The model under review builds one solid part; all positions refer to its coordinate system, in mm. A direction names the side the tool comes from. Round coordinates to 2 decimals unless told otherwise and drop trailing zeros. Order: outer loops, then holes, each group sorted by start corner. A loop starts at its lowest first (then second) coordinate and runs counter-clockwise, first axis right, second up.
Autodesk Inventor part; units mm, degrees
ref_plane "YZ Plane" through (0, 0, 0) normal (1, 0, 0) x (0, 1, 0)
ref_plane "XZ Plane" through (0, 0, 0) normal (0, 1, 0) x (-1, 0, 0)
ref_plane "XY Plane" through (0, 0, 0) normal (0, 0, 1) x (1, 0, 0)
sketch "Sketch1" plane through (0, 0, 0) normal (0, 0, 1) x (1, 0, 0)
  line L0 (-35.56, 0) -> (35.56, 0) construction
  line L1 (0, -35.56) -> (0, 35.56) construction
  line L2 (-25.4, 25.4) -> (25.4, 25.4)
  line L3 (25.4, 25.4) -> (25.4, -25.4)
  line L4 (25.4, -25.4) -> (-25.4, -25.4)
  line L5 (-25.4, -25.4) -> (-25.4, 25.4)
  line L6 (-22.225, 22.225) -> (22.225, 22.225)
  line L7 (22.225, 22.225) -> (22.225, -22.225)
  line L8 (22.225, -22.225) -> (-22.225, -22.225)
  line L9 (-22.225, -22.225) -> (-22.225, 22.225)
  point P0 (0, 0)
  point P1 (-25.4, 0)
  point P2 (0, 25.4)
  point P3 (-22.225, 0)
  point P4 (0, 22.225)
  dimension "d0" = 50.8
  dimension "d1" = 3.175
  dimension "d11" = 50.8
  dimension "d12" = 3.175
extrude "Extrusion1" add sketch "Sketch1" along normal mid plane 101.6
sketch "Sketch6" plane through (-25.4, -25.4, 50.8) normal (-1, 0, 0) x (0, 0, 1)
  circle A0 centre (-68.7605, 43.3605) radius 2.0193 construction
  circle A1 centre (-32.8395, 7.4395) radius 2.0193 construction
  circle A2 centre (-50.8, 25.4) radius 6.985
  line L0 (0, 47.625) -> (-101.6, 47.625) construction
  line L1 (-101.6, 3.175) -> (-101.6, 47.625) construction
  line L2 (0, 3.175) -> (-101.6, 3.175) construction
  line L3 (0, 47.625) -> (0, 3.175) construction
  circle A3 centre (-86.7029, 41.275) radius 3.175
  circle A4 centre (-14.8971, 9.525) radius 3.175
  circle A5 centre (-86.7029, 9.525) radius 3.175
  circle A6 centre (-14.8971, 41.275) radius 3.175
  circle A7 centre (-68.7605, 43.3605) radius 2.413
  circle A8 centre (-32.8395, 7.4395) radius 2.413
  point P0 (-50.8, 25.4)
  dimension "d38" = 4.826
sketch "Sketch7" plane through (25.4, -25.4, 50.8) normal (1, 0, 0) x (0, 0, -1)
  circle A0 centre (50.8, 25.4) radius 14.2875
  dimension "d25" = 28.575
extrude "Extrusion8" cut sketch "Sketch7" against normal up to next
sketch "Sketch8" plane through (-22.225, -22.225, -50.8) normal (1, 0, 0) x (0, 0, -1)
  circle A0 centre (-14.8971, 6.35) radius 2.667
  circle A1 centre (-86.7029, 6.35) radius 2.667
  circle A2 centre (-86.7029, 38.1) radius 2.667
  circle A3 centre (-14.8971, 38.1) radius 2.667
  point P0 (-50.8, 22.225)
extrude "Extrusion9" cut sketch "Sketch8" against normal up to next
sketch "Sketch9" plane through (25.4, -25.4, 50.8) normal (1, 0, 0) x (0, 0, -1)
  circle A0 centre (14.8971, 9.525) radius 3.175
  circle A1 centre (14.8971, 41.275) radius 3.175
  circle A2 centre (86.7029, 9.525) radius 3.175
  circle A3 centre (86.7029, 41.275) radius 3.175
  point P0 (50.8, 25.4)
extrude "Extrusion10" cut sketch "Sketch9" against normal up to next
sketch "Sketch10" plane through (22.225, -22.225, -50.8) normal (-1, 0, 0) x (0, 0, 1)
  circle A0 centre (69.85, 22.225) radius 2.667 construction
  circle A1 centre (31.75, 22.225) radius 2.667 construction
  circle A2 centre (69.85, 22.225) radius 3.175
  circle A3 centre (31.75, 22.225) radius 3.175
  point P0 (50.8, 22.225)
  dimension "d32" = 6.35
extrude "Extrusion11" cut sketch "Sketch10" against normal through all
sketch "Sketch11" plane through (25.4, -25.4, 50.8) normal (1, 0, 0) x (0, 0, -1)
  circle A0 centre (68.7605, 43.3605) radius 2.0193 construction
  circle A1 centre (32.8395, 7.4395) radius 2.0193 construction
  circle A2 centre (68.7605, 43.3605) radius 3.175
  circle A3 centre (32.8395, 7.4395) radius 3.175
  point P0 (50.8, 25.4)
  dimension "d35" = 6.35
extrude "Extrusion12" cut sketch "Sketch11" against normal up to next
extrude "Extrusion13" cut sketch "Sketch6" against normal up to next contours A2 | A7 | A8
equation "\"d12\" = d1"
properties part number "Arm 4 inch" material "Aluminum 6061"
(1) For faces 1 (the cylindrical face through (-23.835, 19.995, -16.663)), 2 (the flat face through (0, 22.225, -1)), 3 (the cylindrical face through (23.83, 18.1, -14.79)), list the 3-axis set-ups (+Z, -Z, +X, -X, +Y, -Y) from which the entire face can be reached by the end or side of a thin tool; tool diameter is ignored.
Data:
face 1: +X, -X
face 2: +Z, -Z
face 3: +X
(2) Consider section B-B (z = 0). Write out the cut boundary in (x, y) (1 decimal), and give its area (3 significant figures).
Data:
outline: (-25.4, -25.4) - (25.4, -25.4) - (25.4, -14.3) - (22.2, -14.3) - (22.2, -22.2) - (-22.2, -22.2) - (-22.2, -7) - (-25.4, -7) - close; (-25.4, 7) - (-22.2, 7) - (-22.2, 22.2) - (22.2, 22.2) - (22.2, 14.3) - (25.4, 14.3) - (25.4, 25.4) - (-25.4, 25.4) - close
area: 470 mm2
(3) Insertion check: pin 1 (7.5 mm diameter, centred on y = 0, z = -19.05, fed in from +X); pin 2 (4 mm diameter, centred on y = 0, z = 19.05, fed in from +X) (3 decimals). Each pin has a flat end and moves straight along its axis. Give the tip position at first contact, or say it passes through.
Data:
pin 1: stops at x = 25.4
pin 2: stops at x = -22.225
(4) Consider section A-A (y = 0). Write out the cut boundary in (x, z) (1 decimal), and give its area (3 significant figures).
Data:
outline: (-25.4, -50.8) - (-22.2, -50.8) - (-22.2, -7) - (-25.4, -7) - close; (-25.4, 7) - (-22.2, 7) - (-22.2, 50.8) - (-25.4, 50.8) - close; (22.2, -50.8) - (25.4, -50.8) - (25.4, -22.2) - (22.2, -22.2) - close; (22.2, -15.9) - (25.4, -15.9) - (25.4, -14.3) - (22.2, -14.3) - close; (22.2, 14.3) - (25.4, 14.3) - (25.4, 15.9) - (22.2, 15.9) - close; (22.2, 22.2) - (25.4, 22.2) - (25.4, 50.8) - (22.2, 50.8) - close
area: 470 mm2
(5) Consider section C-C (x = -21). Write out the cut boundary in (y, z) (3 decimals), and give its area (3 significant figures).
Data:
outline: (-25.4, -50.8) - (-22.225, -50.8) - (-22.225, 50.8) - (-25.4, 50.8) - close; (22.225, -50.8) - (25.4, -50.8) - (25.4, 50.8) - (22.225, 50.8) - close
area: 645 mm2
(6) Consider section D-D (z = 41). Write out the cut boundary in (x, y) (3 decimals), and give its area (3 significant figures).
Data:
outline: (-25.4, -25.4) - (25.4, -25.4) - (25.4, 25.4) - (-25.4, 25.4) - close; hole (-22.225, -22.225) - (22.225, -22.225) - (22.225, 22.225) - (-22.225, 22.225) - close
area: 605 mm2
(7) To check wall thickness, follow probe 1 along X at (y, z) = (13, 30) (3 decimals); probe 2 along Y at (x, z) = (-23.05, 0) (3 decimals). State the ranges of each line that lie inside material, in increasing order.
Data:
probe 1: x = -25.4 to -22.225, 22.225 to 25.4
probe 2: y = -25.4 to -6.985, 6.985 to 25.4
(8) Draft analysis for pull direction Y (two halves, no side actions). For faces 4 (the flat face through (-23, 0, -50.8)), 5 (the cylindrical face through (-23.835, 6.926, -0.909)), 6 (the flat face through (0, -25.4, -1)), state which applies: pulls with the +Y half, pulls with the -Y half, needs draft (parallel to the pull), parting line crosses it, or undercut.
Data:
face 4: needs draft
face 5: undercut
face 6: pulls with the -Y half
